Can you work these out from the model? Positions are in its coordinate system, mm. A direction names the side the tool comes from. Round coordinates to 2 decimals unless told otherwise and drop trailing zeros. Order: outer loops, then holes, each group sorted by start corner. A loop starts at its lowest first (then second) coordinate and runs counter-clockwise, first axis right, second up.
Q1. We'd pull the mould along Y, two halves only. Please class faces 4 (the face through (-276.803, 108.187, 187.302)), 5 (the face through (-12.264, 257.095, -56.503)): pulls with the +Y half, pulls with the -Y half, needs draft (parallel to the pull), parting line crosses it, or undercut.
Q2. Will these pins go through, and if not, where does the flat tip stop? P1, Ø8, axis at x = -127.5, z = -47, coming from the +Y side; P2, Ø21.5, axis at x = -284, y = 22.5, coming from the +Z side; P3, Ø5, axis at x = -34.5, z = -12, coming from the -Y side.
Q3. If I drill on line 1 (Y direction, x = -69.5, z = -88.5); line 2 (Z direction, x = 152, y = -254); line 3 (Z direction, x = -36, y = 253.5), over which ranges is the centre line in solid material (lowest first)?
Q4. If we section it at B-B (z = -142): Please give me the cut outline in (x, y).
Q5. If we section it at A-A (x = 203): Please give me the cut outline in (y, z), plus the area to 3 significant figures.
Q6. For faces 1 (the face through (-153, 253, 177.442)), 2 (the face through (-132.19, 311.42, 189.94)), 3 (the face through (-193.933, -134.862, 33.358)), which set-ups out of +Z, -Z, +X, -X, +Y, -Y let a thin tool reach every point of the face, with its end or its side?
from build123d import *
from build123d.topology import SkipClean

# Parameters (mm, degrees)
BOSS_EXTRUDE1_DEPTH          = 35
SKETCH5_W                    = 110
SKETCH5_H                    = 110
BOSS_EXTRUDE2_DEPTH          = 55
BOSS_EXTRUDE3_DEPTH          = 10
FILLET1_R                    = 20
FILLET4_R                    = 10
SKETCH12_W                   = 221.575141924
SKETCH12_H                   = 185.580798287
CUT_REVOLVE1_ANGLE           = 32
CUT_REVOLVE1_OTHER_WAY_ANGLE = 109
BOSS_EXTRUDE4_REACH          = 690.076
SKETCH15_W                   = 208.026220801
SKETCH15_H                   = 123.720532191
CUT_REVOLVE2_ANGLE           = 20
SKETCH16_W                   = 103.379457842
SKETCH16_H                   = 185.232234629
CUT_REVOLVE3_ANGLE           = 20
SKETCH17_W                   = 90
SKETCH17_H                   = 120
REVOLVE3_ANGLE               = 74
REVOLVE3_OTHER_WAY_ANGLE     = 67
SKETCH18_W                   = 70
SKETCH18_H                   = 100
CUT_REVOLVE4_ANGLE           = 94
SKETCH19_W                   = 306.456266988
SKETCH19_H                   = 205.283587683
REVOLVE4_ANGLE               = 17
SKETCH20_W                   = 69.271583649
SKETCH20_H                   = 57.641793842
REVOLVE5_ANGLE               = 10
REVOLVE6_ANGLE               = 45
REVOLVE7_ANGLE               = 33
BOSS_EXTRUDE5_DEPTH          = 20
CIRPATTERN1_COUNT            = 5
CIRPATTERN1_ANGLE            = 62.64


with BuildPart() as part:
    # Sketch4 → Boss-Extrude1 (new body)
    with BuildSketch(Plane.XY.offset(90)):
        with BuildLine():
            ThreePointArc((18, 0), (12.727922061, 12.727922061), (0, 18))
            Line((0, 18), (-40, 18))
            Line((-40, 18), (-40, 0))
            Line((-40, 0), (-5, 0))
            ThreePointArc((-5, 0), (0, 5), (5, 0))
            Line((5, 0), (18, 0))
        make_face()
        with BuildLine():
            ThreePointArc((0, -18), (12.727922061, -12.727922061), (18, 0))
            Line((18, 0), (5, 0))
            ThreePointArc((5, 0), (0, -5), (-5, 0))
            Line((-5, 0), (-40, 0))
            Line((-40, 0), (-40, -18))
            Line((-40, -18), (0, -18))
        make_face()
    extrude(amount=-BOSS_EXTRUDE1_DEPTH)

    # Sketch5 → Boss-Extrude2 (add)
    with BuildSketch(Plane(origin=(0, 0, 55), x_dir=(-1, 0, 0), z_dir=(0, 0, -1))):
        with Locations((22, 0)):
            Rectangle(SKETCH5_W, SKETCH5_H)
    extrude(amount=BOSS_EXTRUDE2_DEPTH)

    # Sketch7 → Boss-Extrude3 (add)
    with BuildSketch(Plane(origin=(0, 0, 0), x_dir=(-1, 0, 0), z_dir=(0, 0, -1))):
        Polygon((87, -65), (125, -79.925557452), (125, 79.925557452), (87, 65), (-43, 65), (-43, -65), align=None)
    extrude(amount=-BOSS_EXTRUDE3_DEPTH)

    # Fillet1
    fillet1_edges = [part.edges().sort_by_distance(p)[0] for p in [
        (-125, -79.925557452, 5),
        (-87, -65, 5),
        (43, -65, 5),
        (43, 65, 5),
        (-87, 65, 5),
        (-125, 79.925557452, 5),
    ]]
    fillet(fillet1_edges, radius=FILLET1_R)

    # Fillet4
    fillet4_edges = [part.edges().sort_by_distance(p)[0] for p in [
        (-40, -18, 72.5),
        (-40, 18, 72.5),
        (33, 0, 55),
        (-22, -55, 55),
        (-77, 0, 55),
        (-22, 55, 55),
        (33, -55, 32.5),
        (33, 55, 32.5),
        (33, 0, 10),
        (-77, -55, 32.5),
        (-77, 55, 32.5),
        (-77, 0, 10),
        (-22, 55, 10),
        (-22, -55, 10),
    ]]
    fillet(fillet4_edges, radius=FILLET4_R - 0.0001)  # a hair under: the kernel refuses the full size


with BuildPart() as body_2:
    # Sketch8 → Revolve1 (revolve)
    with BuildSketch(Plane(origin=(0, 0, 0), x_dir=(1, 0, 0), z_dir=(0, 1, 0))):
        with BuildLine():
            Line((0, -474), (0, 204))
            ThreePointArc((0, 204), (339, -135), (0, -474))
        make_face()
    revolve(axis=Axis((0, 0, 474), (0, 0, -1)))


with BuildPart() as body_3:
    # Sketch9 → Revolve2 (revolve)
    with BuildSketch(Plane(origin=(0, 0, 0), x_dir=(0, 0, -1), z_dir=(1, 0, 0)), mode=Mode.PRIVATE) as revolve2_sk:
        with BuildLine():
            Line((0, 0), (0, -93.287808854))
            Line((0, -93.287808854), (132.583470884, -93.287808854))
            Line((132.583470884, -93.287808854), (132.583470884, -141.122377334))
            ThreePointArc((132.583470884, -141.122377334), (51.419403359, -224.141377396), (-52.997327403, -274.904617695))
            Line((-52.997327403, -274.904617695), (-52.997327403, -352.684487381))
            Line((-52.997327403, -352.684487381), (204, -352.684487381))
            Line((204, -352.684487381), (204, 0))
            Line((204, 0), (0, 0))
        make_face()
    revolve(revolve2_sk.sketch.rotate(Axis((0, 0, 0), (0, 0, -1)), 270), axis=Axis((0, 0, 0), (0, 0, -1)))

    # Sketch12 → Cut-Revolve1 (revolve, cut)
    with BuildSketch(Plane(origin=(0, 0, 0), x_dir=(1, 0, 0), z_dir=(0, 1, 0))):
        with Locations((241.896916419, 39.793071741)):
            Rectangle(SKETCH12_W, SKETCH12_H)
    revolve(axis=Axis((0, 0, 0), (0, 0, -1)), revolution_arc=CUT_REVOLVE1_ANGLE, mode=Mode.SUBTRACT)

    # Sketch12 → Cut-Revolve1 other way (revolve, cut)
    with BuildSketch(Plane(origin=(0, 0, 0), x_dir=(1, 0, 0), z_dir=(0, 1, 0))):
        with Locations((241.896916419, 39.793071741)):
            Rectangle(SKETCH12_W, SKETCH12_H)
    revolve(axis=Axis((0, 0, 0), (0, 0, 1)), revolution_arc=CUT_REVOLVE1_OTHER_WAY_ANGLE, mode=Mode.SUBTRACT)

    # Sketch14 → Boss-Extrude4 (add, up to next)
    with BuildSketch(Plane.XY, mode=Mode.PRIVATE) as boss_extrude4_sk1:
        with BuildLine():
            Line((19.076881684, -91.316416191), (-234.050666272, -144.197206796))
            ThreePointArc((-234.050666272, -144.197206796), (-274.904617695, 0), (-234.050666272, 144.197206796))
            Line((-234.050666272, 144.197206796), (19.076881684, 91.316416191))
            ThreePointArc((19.076881684, 91.316416191), (93.287808854, 0), (19.076881684, -91.316416191))
        make_face()
    boss_extrude4_tool1 = extrude(boss_extrude4_sk1.sketch, amount=-BOSS_EXTRUDE4_REACH, mode=Mode.PRIVATE) - body_3.part
    add(boss_extrude4_tool1.solids().sort_by_distance((-108.886341, 0, 0))[0])

    # Sketch15 → Cut-Revolve2 (revolve, cut)
    with BuildSketch(Plane(origin=(0, 0, 0), x_dir=(0.8480480961564173, -0.5299192642332188, 0), z_dir=(0.5299192642332188, 0.8480480961564173, 0))):
        with Locations((248.67137698, 8.862938693)):
            Rectangle(SKETCH15_W, SKETCH15_H)
    revolve(axis=Axis((0, 0, 0), (0, 0, -1)), revolution_arc=CUT_REVOLVE2_ANGLE, mode=Mode.SUBTRACT)

    # Sketch16 → Cut-Revolve3 (revolve, cut)
    with BuildSketch(Plane(origin=(0, 0, 0), x_dir=(0, 0, -1), z_dir=(0.7880107536067323, 0.6156614753256451, 0))):
        with Locations((-42.826790228, -260.068370066)):
            Rectangle(SKETCH16_W, SKETCH16_H)
    revolve(axis=Axis((0, 0, 0), (0, 0, -1)), revolution_arc=CUT_REVOLVE3_ANGLE, mode=Mode.SUBTRACT)



with BuildPart() as body_4:
    # Sketch17 → Revolve3 (revolve)
    with BuildSketch(Plane(origin=(0, 0, 0), x_dir=(1, 0, 0), z_dir=(0, 1, 0))):
        with Locations((-307.684487381, -217.442198662)):
            Rectangle(SKETCH17_W, SKETCH17_H)
    revolve(axis=Axis((0, 0, 0), (0, 0, 1)), revolution_arc=REVOLVE3_ANGLE)

    # Sketch17 → Revolve3 other way (revolve)
    with BuildSketch(Plane(origin=(0, 0, 0), x_dir=(1, 0, 0), z_dir=(0, 1, 0))):
        with Locations((-307.684487381, -217.442198662)):
            Rectangle(SKETCH17_W, SKETCH17_H)
    revolve(axis=Axis((0, 0, 0), (0, 0, -1)), revolution_arc=REVOLVE3_OTHER_WAY_ANGLE)

    # Sketch18 → Cut-Revolve4 (revolve, cut)
    with BuildSketch(Plane(origin=(0, 0, 0), x_dir=(0.3907311284892735, -0.9205048534524405, 0), z_dir=(0.9205048534524405, 0.3907311284892735, 0))):
        with Locations((-297.684487381, -227.442198662)):
            Rectangle(SKETCH18_W, SKETCH18_H)
    revolve(axis=Axis((0, 0, 0), (0, 0, 1)), revolution_arc=CUT_REVOLVE4_ANGLE, mode=Mode.SUBTRACT)


with BuildPart() as body_3_1:
    with SkipClean():  # the faces are left unmerged after this step: merging them gives an invalid solid
        add(body_3.part)

        add(body_4.part)  # Revolve4 merges body 4
        # Sketch19 → Revolve4 (revolve)
        with BuildSketch(Plane(origin=(0, 0, 0), x_dir=(0, 0, -1), z_dir=(0.9612616959383228, -0.2756373558169854, 0))):
            with Locations((-4.214065168, -250.04269354)):
                Rectangle(SKETCH19_W, SKETCH19_H)
        revolve(axis=Axis((0, 0, 0), (0, 0, -1)), revolution_arc=REVOLVE4_ANGLE)

    # Sketch20 → Cut-Revolve5 (revolve, cut)
    with SkipClean():  # the faces are left unmerged after this step: merging them gives an invalid solid
        with BuildSketch(Plane(origin=(0, 0, 0), x_dir=(0, 0, -1), z_dir=(0.9612616959383229, -0.27563735581698545, 0)), mode=Mode.PRIVATE) as cut_revolve5_sk:
            with Locations((-122.806406838, -176.221796619)):
                Rectangle(SKETCH20_W, SKETCH20_H)
        revolve(cut_revolve5_sk.sketch.rotate(Axis((0, 0, 0), (0, 0, 1)), 286), axis=Axis((0, 0, 0), (0, 0, 1)), mode=Mode.SUBTRACT)

    # Sketch21 → Revolve5 (revolve)
    with SkipClean():  # the faces are left unmerged after this step: merging them gives an invalid solid
        with BuildSketch(Plane(origin=(0, 0, 0), x_dir=(0.8910065241883608, 0.4539904997395606, 0), z_dir=(-0.4539904997395606, 0.8910065241883608, 0))):
            Polygon((-352.684487381, -177.442198662), (-262.684487381, -177.442198662), (-226.3635331, -200.635504694), (-226.3635331, -369.727899201), (-352.684487381, -369.727899201), align=None)
        revolve(axis=Axis((0, 0, 0), (0, 0, 1)), revolution_arc=REVOLVE5_ANGLE)

    # Sketch23 → Revolve6 (revolve)
    with SkipClean():  # the faces are left unmerged after this step: merging them gives an invalid solid
        with BuildSketch(Plane(origin=(0, 0, 0), x_dir=(0, 0, 1), z_dir=(-0.838670567945428, 0.5446390350150208, 0))):
            with BuildLine():
                Line((52.997327403, -274.904617695), (77.16647828, -274.904617695))
                Line((77.16647828, -274.904617695), (77.16647828, -236.215399807))
                Line((77.16647828, -236.215399807), (-33.492204466, -236.215399807))
                ThreePointArc((-33.492204466, -236.215399807), (8.394219656, -258.596574335), (52.997327403, -274.904617695))
            make_face()
        revolve(axis=Axis((0, 0, 0), (0, 0, -1)), revolution_arc=REVOLVE6_ANGLE)

    # Sketch24 → Revolve7 (revolve)
    with SkipClean():  # the faces are left unmerged after this step: merging them gives an invalid solid
        with BuildSketch(Plane(origin=(0, 0, 0), x_dir=(0, 0, -1), z_dir=(0.9455185755993164, 0.3255681544571581, 0))):
            with BuildLine():
                Line((29.947951331, 238.411319514), (29.947951331, 257.387120756))
                Line((29.947951331, 257.387120756), (82.325244386, 257.387120756))
                Line((82.325244386, 257.387120756), (82.325244386, 352.684487381))
                Line((82.325244386, 352.684487381), (132.583470884, 352.684487381))
                Line((132.583470884, 352.684487381), (132.583470884, 141.122377334))
                ThreePointArc((132.583470884, 141.122377334), (86.395300565, 195.178337821), (29.947951331, 238.411319514))
            make_face()
        revolve(axis=Axis((0, 0, 0), (0, 0, -1)), revolution_arc=REVOLVE7_ANGLE)

    # Sketch25 → Boss-Extrude5 (add)
    with SkipClean():  # the faces are left unmerged after this step: merging them gives an invalid solid
        with BuildSketch(Plane.XY.offset(177.442198662)):
            with BuildLine():
                Line((-324.592860019, -72.927658462), (-256.207891235, -57.971168522))
                ThreePointArc((-256.207891235, -57.971168522), (-257.559046392, -51.637946631), (-258.753675036, -45.273342779))
                Line((-258.753675036, -45.273342779), (-327.618959516, -57.834120637))
                ThreePointArc((-327.618959516, -57.834120637), (-326.193222042, -65.398394765), (-324.592860019, -72.927658462))
            make_face()
        boss_extrude5 = extrude(amount=BOSS_EXTRUDE5_DEPTH)

    # CirPattern1: Boss-Extrude5 ×5 about axis
    cirpattern1_axis = Axis((0, 0, 0), (0, 0, -1))
    for i in range(1, CIRPATTERN1_COUNT):
        add(boss_extrude5.rotate(cirpattern1_axis, i * CIRPATTERN1_ANGLE / (CIRPATTERN1_COUNT - 1)))


solid = body_3_1.part
Solution:
1. face 4: undercut
1. face 5: pulls with the +Y half
2. P1: stops at y = 330.35
2. P2: stops at z = 197.44
2. P3: stops at y = -351.23
3. line 1: y = -345.77 to -129.99, -109.82 to 109.82, 180.23 to 345.77
3. line 2: z = -204 to -8.86
3. line 3: z = -204 to -29.95
4. outline: circle Ø705.37 at (0, 0)
5. outline: (-288.4, -204) - (288.4, -204) - (288.4, -132.58) - (-126.85, -132.58) - (-126.85, -70.72) - (-259.83, -70.72) - (-259.83, -8.86) - (-288.4, -8.86) - close
5. area: 53,000 mm2
6. face 1: +Z, +X
6. face 2: +Z, +X, +Y
6. face 3: none
